Build history of the part. All positions in model axes, mm. Face numbers are marked on the shaded views. A direction names the side the tool comes from. Coordinates: 2 decimals unless noted, no trailing zeros. Loops run counter-clockwise (first coordinate to the right, second up) from the corner with the lowest first, then second, coordinate; pieces in that order, holes last.
(1) Slice it at B-B (y = 60). Give the cut face in (x, z), and give its area (3 significant figures).
(2) Slice it at C-C (y = 73). Give the cut face in (x, z), and give its area (3 significant figures).
(3) Flat gauge pins, fed straight in: P1, Ø12, axis at y = 31.5, z = 20, coming from the +X side; P2, Ø19, axis at x = -36.59, y = 14.92, coming from the -Z side; P3, Ø21, axis at x = -25.5, y = 32.5, coming from the +Z side. Where does each tip first touch, or does it go through?
(4) Slice it at A-A (x = 20.5). Give the cut face in (y, z), and give its area (3 significant figures).
(5) Tool access for the marked faces 4 and 5: list every direction of +Z, -Z, +X, -X, +Y, -Y with a clear straight run to the whole face (end or side of a thin tool).
(6) Wall check: L1, parallel to Z at x = -25.5, y = 42; L2, parallel to Y at x = -32, z = -15; L3, parallel to Z at x = 3, y = 49.5. Give the ranges that are in metal, low to high.
(7) Two-plate mould, pull along Z, no slides. Class the marked faces 1, 2 and 3: pulls with the +Z half, pulls with the -Z half, needs draft (parallel to the pull), parting line crosses it, or undercut.
from build123d import *

# Parameters (mm, degrees)
SKETCH1_R               = 26.5
SKETCH1_R_2             = 22.5
BOSS_EXTRUDE1_DEPTH     = 82
SKETCH3_W               = 52
SKETCH3_H               = 49
BOSS_EXTRUDE2_DEPTH     = 80
CUT_EXTRUDE1_DEPTH      = 101.649143066
CUT_EXTRUDE1_DEPTH_BACK = 101.649143066
SHELL1_DEPTH            = 76
CUT_EXTRUDE2_START      = -80
CUT_EXTRUDE2_DEPTH      = 80
FILLET1_R               = 15.409961
FILLET2_R               = 15.409961
SKETCH6_R               = 6
CUT_EXTRUDE3_DEPTH      = 80


# Read off the part's stored shape, not the designer's step: Shell1
with BuildPart() as part:
    # Sketch1 → Boss-Extrude1 (new body)
    with BuildSketch(Plane(origin=(0, 0, 0), x_dir=(1, 0, 0), z_dir=(0, 1, 0))):
        with Locations(Location((0, 0, 0), (0, 0, 270))):
            Circle(SKETCH1_R)
        with Locations(Location((0, 0, 0), (0, 0, 270))):
            Circle(SKETCH1_R_2, mode=Mode.SUBTRACT)
    extrude(amount=BOSS_EXTRUDE1_DEPTH)

    # Sketch3 → Boss-Extrude2 (add)
    with BuildSketch(Plane(origin=(0, 0, 0), x_dir=(1, 0, 0), z_dir=(0, 1, 0))):
        with Locations((-26, 0)):
            Rectangle(SKETCH3_W, SKETCH3_H)
    extrude(amount=BOSS_EXTRUDE2_DEPTH)

    # Sketch4 → Cut-Extrude1 (cut, two sides: drawn at the far end of the back side and taken through both)
    with BuildSketch(Plane.XY.offset(-CUT_EXTRUDE1_DEPTH_BACK)):
        Polygon((163.095245714, 245.965543737), (26.5, 71.131601988), (-29.074098223, 0), (-165.669343938, -174.833941749), (183.998539561, -448.024433177), (512.763129212, -27.224947691), align=None)
    extrude(amount=CUT_EXTRUDE1_DEPTH + CUT_EXTRUDE1_DEPTH_BACK, mode=Mode.SUBTRACT)

    # Shell1 outline → Shell1 (cut)
    with BuildSketch(Plane(origin=(0, 0, 0), x_dir=(1, 0, 0), z_dir=(0, 1, 0))):
        with BuildLine():
            ThreePointArc((-9.273618496, -20.5), (-6.687371777, -21.483227381), (-4, -22.141589825))
            Line((-4, -22.141589825), (-4, 22.141589825))
            ThreePointArc((-4, 22.141589825), (-6.687371776, 21.483227381), (-9.273618495, 20.5))
            Line((-9.273618495, 20.5), (-52, 20.5))
            Line((-52, 20.5), (-52, -20.5))
            Line((-52, -20.5), (-9.273618496, -20.5))
        make_face()
    extrude(amount=SHELL1_DEPTH, mode=Mode.SUBTRACT)

    # Sketch5 → Cut-Extrude2 (cut)
    with BuildSketch(Plane(origin=(0, 80, 0), x_dir=(1, 0, 0), z_dir=(0, 1, 0)).offset(CUT_EXTRUDE2_START)):
        with BuildLine():
            Line((0, -22.5), (0, 22.5))
            ThreePointArc((0, 22.5), (-22.5, 0), (0, -22.5))
        make_face()
    extrude(amount=CUT_EXTRUDE2_DEPTH, mode=Mode.SUBTRACT)

    # Fillet1
    fillet1_edges = [part.edges().sort_by_distance(p)[0] for p in [
        (-52, 0, -22.5),
        (-29.074098223, 0, -22.5),
    ]]
    fillet(fillet1_edges, radius=FILLET1_R)

    # Fillet2
    fillet2_edges = [part.edges().sort_by_distance(p)[0] for p in [
        (-29.074098223, 0, 22.5),
        (-52, 0, 22.5),
    ]]
    fillet(fillet2_edges, radius=FILLET2_R)

    # Sketch6 → Cut-Extrude3 (cut)
    with BuildSketch(Plane.XY.offset(24.5)):
        with Locations((-36.590038591, 14.924477303)):
            Circle(SKETCH6_R)
    extrude(amount=-CUT_EXTRUDE3_DEPTH, mode=Mode.SUBTRACT)


solid = part.part
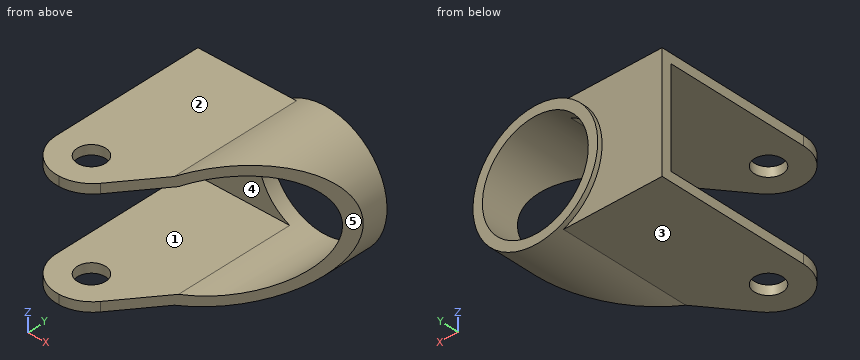
Response values:
1. outline: (-52, -24.5) - (-10.1, -24.5) arc R26.5 ccw to (17.8, -19.63) - (17.8, -13.76) arc R22.5 cw to (-9.27, -20.5) - (-52, -20.5) - close; (-52, 20.5) - (-9.27, 20.5) arc R22.5 cw to (17.8, 13.76) - (17.8, 19.63) arc R26.5 ccw to (-10.1, 24.5) - (-52, 24.5) - close
1. area: 578 mm2
2. outline: (-52, -24.5) - (-10.1, -24.5) arc R26.5 ccw (long way) to (-10.1, 24.5) - (-52, 24.5) - (-52, 20.5) - (-9.27, 20.5) arc R22.5 cw (long way) to (-9.27, -20.5) - (-52, -20.5) - close
2. area: 726 mm2
3. P1: stops at x = -0.2
3. P2: stops at z = -24.5
3. P3: stops at z = 24.5
4. outline: (63.45, -16.79) - (82, -16.79) - (82, -9.27) - (63.45, -9.27) - close; (63.45, 9.27) - (82, 9.27) - (82, 16.79) - (63.45, 16.79) - close
4. area: 279 mm2
5. face 4: -X, -Y
5. face 5: +Z, -Z, +X, -Y
6. L1: z = -24.5 to -20.5, 20.5 to 24.5
6. L2: y = 76 to 80
6. L3: z = -26.33 to -22.3, 22.3 to 26.33
7. face 1: undercut
7. face 2: pulls with the +Z half
7. face 3: pulls with the -Z half
